from build123d import *

# Parameters (mm, degrees)
F0_R     = 19
F0_R_2   = 13
F1_DEPTH = 4
F2_SIZE  = 1
F3_SIZE  = 2
F5_DEPTH = 4.001


with BuildPart() as f1:
    # F0 (on Top) → F1 (new body)
    with BuildSketch(Plane.XY):
        Circle(F0_R)
        Circle(F0_R_2, mode=Mode.SUBTRACT)
    extrude(amount=-F1_DEPTH)

    # F2
    f2_edges = [f1.edges().sort_by_distance(p)[0] for p in [
        (-19, 0, 0),
    ]]
    chamfer(f2_edges, length=F2_SIZE)

    # F3
    f3_edges = [f1.edges().sort_by_distance(p)[0] for p in [
        (-13, 0, 0),
    ]]
    chamfer(f3_edges, length=F3_SIZE)

    # F4 (on face) → F5 (cut, through all)
    with BuildSketch(Plane.XY):
        with BuildLine():
            Line((-1, 18.973666), (-1, 18))
            Line((-1, 18), (1, 18))
            Line((1, 18), (1, 18.973666))
            ThreePointArc((1, 18.973666), (0, 19), (-1, 18.973666))
        make_face()
        with BuildLine():
            Line((1, -18), (-1, -18))
            Line((-1, -18), (-1, -18.973666))
            ThreePointArc((-1, -18.973666), (0, -19), (1, -18.973666))
            Line((1, -18.973666), (1, -18))
        make_face()
    extrude(amount=-F5_DEPTH, mode=Mode.SUBTRACT)


solid = f1.part
Build history of the part. All positions in model axes, mm. A direction names the side the tool comes from. Coordinates: 2 decimals unless noted, no trailing zeros. Write each loop counter-clockwise with the first axis right and the second up, starting at its lowest first coordinate (ties: lowest second). Pieces come first, ordered by that corner, then holes.
(1) Cut at A-A on y = 0. List the corners of the cut face in (x, z), and give its area (3 significant figures).
(2) Drill centre lines: line 1 (Y direction, x = 0, z = -2.7); line 2 (X direction, y = -3, z = -3.6); line 3 (X direction, y = 3, z = -0.55). Where is each one in solid material? Low to high.
(3) Pin check, flat tips, straight feed: pin 1 Ø1.6 at (x, z) = (-0.5, -2.5) entering from +Y; pin 2 Ø1.5 at (x, z) = (-6, -1.5) entering from -Y. Stop position of each tip, or through.
(4) 3-axis set-ups, long thin cutter, end or side, ignore diameter. For faces 5 (the flat face through (-1, -18.5, -2.4)), 6 (the flat face through (-1, 18.5, -2.4)), 7 (the flat face through (-4, 15, 0)): which of +Z, -Z, +X, -X, +Y, -Y reach the whole face in a straight line?
(5) Mould opens along Y. For faces 1 (the flat face through (0, -18, -2)), 2 (the flat face through (1, 18.5, -2.4)), 3 (the conical face through (18.155, -0.399, -0.16)), 4 (the cylindrical face through (-10.316, -7.91, -2.986)) say: pulls with the +Y half, pulls with the -Y half, needs draft (parallel to the pull), parting line crosses it, or undercut.
Working result:
1. outline: (-19, -4) - (-13, -4) - (-13, -2) - (-15, 0) - (-18, 0) - (-19, -1) - close; (13, -4) - (19, -4) - (19, -1) - (18, 0) - (15, 0) - (13, -2) - close
1. area: 43.0 mm2
2. line 1: y = -18 to -13, 13 to 18
2. line 2: x = -18.76 to -12.65, 12.65 to 18.76
2. line 3: x = -18.31 to -14.14, 14.14 to 18.31
3. pin 1: stops at y = 18.97
3. pin 2: stops at y = -18.26
4. face 5: +Z, -Z, -Y
4. face 6: +Z, -Z, +Y
4. face 7: +Z, +X, -X, +Y, -Y
5. face 1: pulls with the -Y half
5. face 2: needs draft
5. face 3: parting line crosses it
5. face 4: undercut
